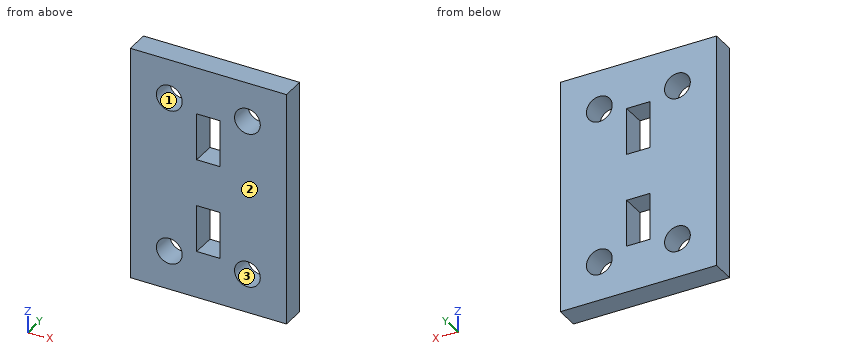
```python
from build123d import *

# Parameters (mm, degrees)
SKETCH1_W           = 20
SKETCH1_H           = 30
SKETCH1_R           = 1.65
SKETCH1_W_2         = 3
SKETCH1_H_2         = 6
BOSS_EXTRUDE1_DEPTH = 3


with BuildPart() as part:
    # Sketch1 → Boss-Extrude1 (new body)
    with BuildSketch(Plane(origin=(0, 0, 0), x_dir=(1, 0, 0), z_dir=(0, 1, 0))):
        Rectangle(SKETCH1_W, SKETCH1_H)
        with Locations((-5, -10)):
            Circle(SKETCH1_R, mode=Mode.SUBTRACT)
        with Locations((5, -10)):
            Circle(SKETCH1_R, mode=Mode.SUBTRACT)
        with Locations((5, 10)):
            Circle(SKETCH1_R, mode=Mode.SUBTRACT)
        with Locations((-5, 10)):
            Circle(SKETCH1_R, mode=Mode.SUBTRACT)
        with Locations((0, 6)):
            Rectangle(SKETCH1_W_2, SKETCH1_H_2, mode=Mode.SUBTRACT)
        with Locations((0, -6)):
            Rectangle(SKETCH1_W_2, SKETCH1_H_2, mode=Mode.SUBTRACT)
    extrude(amount=BOSS_EXTRUDE1_DEPTH)


solid = part.part
```
Verification items for the finished model (mm, model axes). Face numbers are marked on the shaded views. Round coordinates to 2 decimals unless told otherwise and drop trailing zeros. Write each loop counter-clockwise with the first axis right and the second up, starting at its lowest first coordinate (ties: lowest second). Pieces come first, ordered by that corner, then holes.
1. Section check D-D on z = -10. Enter the section's corners in (x, y), plus the area to 3 significant figures.
2. Section check A-A on x = 5. Enter the section's corners in (y, z), plus the area to 3 significant figures.
3. Section check C-C on y = 2.2. Enter the section's corners in (x, z), plus the area to 3 significant figures.
4. Section check B-B on z = -5.25. Enter the section's corners in (x, y), plus the area to 3 significant figures.
5. Scan lines: L1, parallel to Z at x = 5, y = 1.6; L2, parallel to X at y = 1, z = 10; L3, parallel to Z at x = 0.75, y = 1.75. Record each from-to range of solid material in increasing order.
6. Draft check along Z on the marked faces 1, 2 and 3. Enter one of: +Z half, -Z half, draft (parallel to the pull), parting line (faces both ways), or undercut.
Answer:
1. outline: (-10, 0) - (-6.65, 0) - (-6.65, 3) - (-10, 3) - close; (-3.35, 0) - (3.35, 0) - (3.35, 3) - (-3.35, 3) - close; (6.65, 0) - (10, 0) - (10, 3) - (6.65, 3) - close
1. area: 40.2 mm2
2. outline: (0, -15) - (3, -15) - (3, -11.65) - (0, -11.65) - close; (0, -8.35) - (3, -8.35) - (3, 8.35) - (0, 8.35) - close; (0, 11.65) - (3, 11.65) - (3, 15) - (0, 15) - close
2. area: 70.2 mm2
3. outline: (-10, -15) - (10, -15) - (10, 15) - (-10, 15) - close; hole circle Ø3.3 at (-5, -10); hole circle Ø3.3 at (-5, 10); hole (-1.5, -9) - (1.5, -9) - (1.5, -3) - (-1.5, -3) - close; hole (-1.5, 3) - (1.5, 3) - (1.5, 9) - (-1.5, 9) - close; hole circle Ø3.3 at (5, -10); hole circle Ø3.3 at (5, 10)
3. area: 530 mm2
4. outline: (-10, 0) - (-1.5, 0) - (-1.5, 3) - (-10, 3) - close; (1.5, 0) - (10, 0) - (10, 3) - (1.5, 3) - close
4. area: 51.0 mm2
5. L1: z = -15 to -11.65, -8.35 to 8.35, 11.65 to 15
5. L2: x = -10 to -6.65, -3.35 to 3.35, 6.65 to 10
5. L3: z = -15 to -9, -3 to 3, 9 to 15
6. face 1: undercut
6. face 2: draft
6. face 3: undercut
